Input: dimensioned drawing with shaded views. Units: mm. Origin: part minimum x, y, z. Coordinates: 2 decimals unless noted, no trailing zeros. Loops run counter-clockwise (first coordinate to the right, second up) from the corner with the lowest first, then second, coordinate; pieces in that order, holes last.
(1) Section A-A, the plane y = 4.7. Return loops of the section in (x, z).
(2) Section C-C, the plane x = 18. Return loops of the section in (y, z) (1 decimal).
(3) Line query: L1, parallel to Z at x = 18.25, y = 5.2 (1 decimal); L2, parallel to Y at x = 8.5, z = 5; L3, parallel to X at y = 2.2, z = 17 (1 decimal). Output: solid intervals per line, ascending.
(4) Section B-B, the plane x = 10. Return loops of the section in (y, z).
(5) Section D-D, the plane y = 2.2. Return loops of the section in (x, z).
(6) Contact query for flat-ended pins moving along their axis: P1, Ø1.5, axis at y = 3.5, z = 14.5, coming from the -X side; P2, Ø6, axis at x = 13, z = 12.5, coming from the -Y side; P3, Ø3, axis at y = 3.5, z = 20, coming from the -X side. Output: stop coordinate, or through.
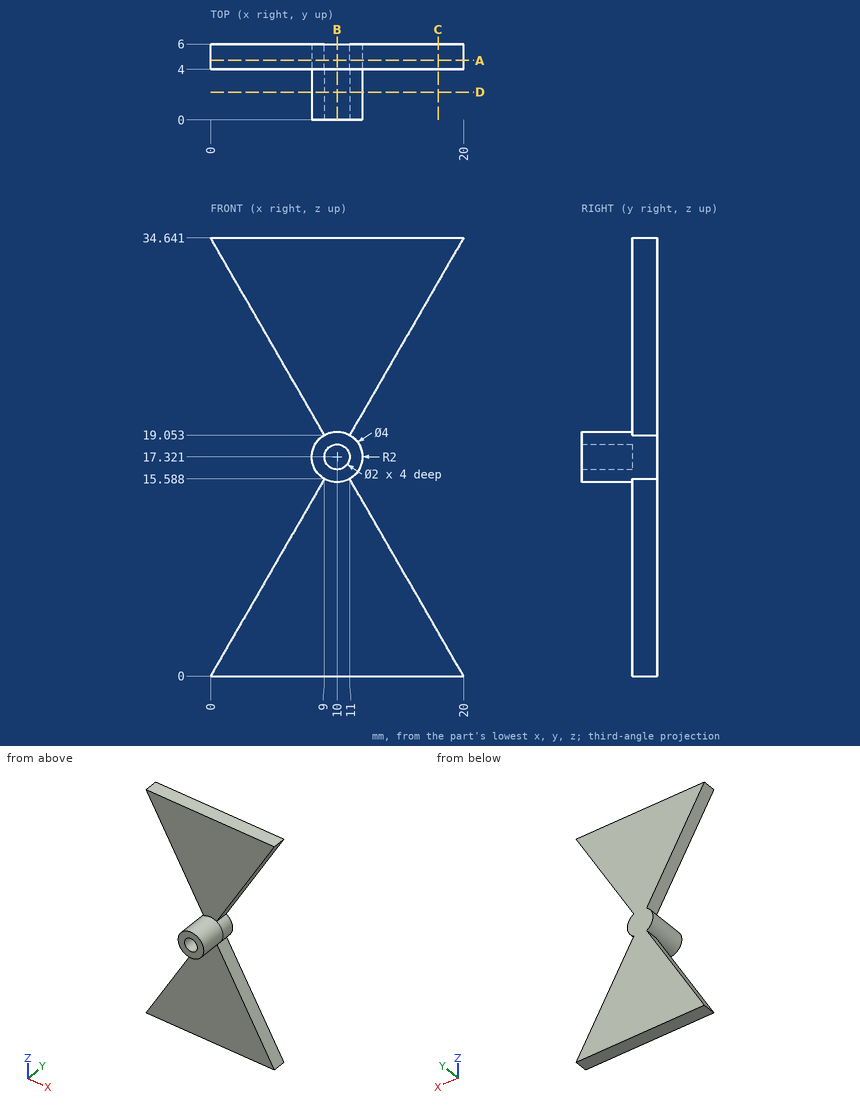
Report:
1. outline: (0, 0) - (20, 0) - (11, 15.59) arc R2 ccw to (11, 19.05) - (20, 34.64) - (0, 34.64) - (9, 19.05) arc R2 ccw to (9, 15.59) - close
2. outline: (4, 0) - (6, 0) - (6, 3.5) - (4, 3.5) - close; (4, 31.2) - (6, 31.2) - (6, 34.6) - (4, 34.6) - close
3. L1: z = 0 to 3, 31.6 to 34.6
3. L2: y = 4 to 6
3. L3: x = 8 to 9.1, 10.9 to 12
4. outline: (0, 15.32) - (4, 15.32) - (4, 0) - (6, 0) - (6, 34.64) - (4, 34.64) - (4, 19.32) - (0, 19.32) - (0, 18.32) - (4, 18.32) - (4, 16.32) - (0, 16.32) - close
5. outline: circle Ø4 at (10, 17.32); hole circle Ø2 at (10, 17.32)
6. P1: stops at x = 8.05
6. P2: stops at y = 4
6. P3: stops at x = 7.64
